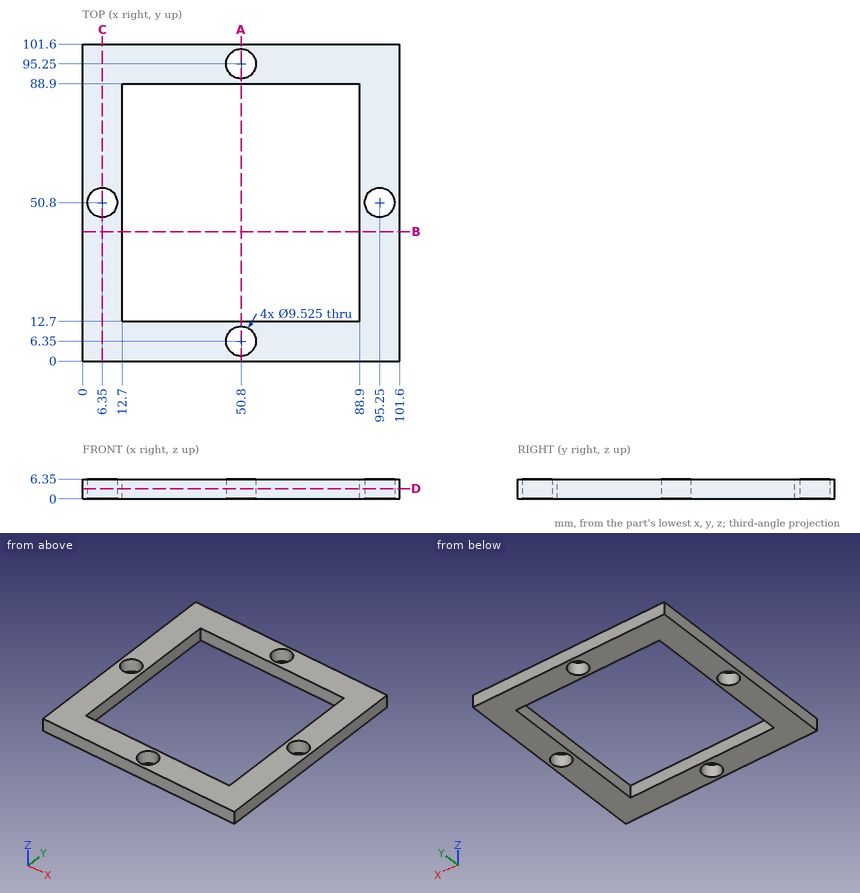
Could you check a few things on this drawing? It's one solid part, dimensions in mm from its lowest x, y, z. Coordinates: 2 decimals unless noted, no trailing zeros. Loops run counter-clockwise (first coordinate to the right, second up) from the corner with the lowest first, then second, coordinate; pieces in that order, holes last. Notation, with made-up numbers: (78.5, -7.5) - (124.5, -7.5) arc R22 cw to (124.5, 16.5) - close; hole circle Ø1 at (-20.5, 43.5). An arc over 180 degrees is marked (long way). Return JSON: item names as keys, results as strings. Group by question number.
Item 1: If we section it at A-A on x = 50.8: Write out the boundary of the cut face in (y, z), and give its area (3 significant figures).
Item 2: If we section it at C-C on x = 6.35: Write out the boundary of the cut face in (y, z), and give its area (3 significant figures).
Item 3: If we section it at B-B on y = 41.5: Write out the boundary of the cut face in (x, z), and give its area (3 significant figures).
Item 4: If we section it at D-D on z = 3.25: State how many separate pieces and enclosed holes the cut face has, and give its area (3 significant figures).
Item 5: Will this pin go through, and if not, where does the flat tip stop? P1, Ø5.5, axis at x = 50.8, y = 6.35, coming from the -Z side.
Item 6: I need wall thicknesses on line 1 (Y direction, x = 50.8, z = 4.5); line 2 (Y direction, x = 6.35, z = 2.25); line 3 (X direction, y = 44, z = 2.25). Which ranges of each line are inside material? Lowest first, please. Write a range as from..to.
Calculated:
{
 "1": {"outline": "(0, 0) - (1.59, 0) - (1.59, 6.35) - (0, 6.35) - close; (11.11, 0) - (12.7, 0) - (12.7, 6.35) - (11.11, 6.35) - close; (88.9, 0) - (90.49, 0) - (90.49, 6.35) - (88.9, 6.35) - close; (100.01, 0) - (101.6, 0) - (101.6, 6.35) - (100.01, 6.35) - close", "area": "40.3 mm^2"},
 "2": {"outline": "(0, 0) - (46.04, 0) - (46.04, 6.35) - (0, 6.35) - close; (55.56, 0) - (101.6, 0) - (101.6, 6.35) - (55.56, 6.35) - close", "area": "585 mm^2"},
 "3": {"outline": "(0, 0) - (12.7, 0) - (12.7, 6.35) - (0, 6.35) - close; (88.9, 0) - (101.6, 0) - (101.6, 6.35) - (88.9, 6.35) - close", "area": "161 mm^2"},
 "4": {"separate pieces": "1", "enclosed holes": "5", "area": "4,230 mm^2"},
 "5": {"P1": "passes through"},
 "6": {"line 1": "y = 0..1.59, 11.11..12.7, 88.9..90.49, 100.01..101.6", "line 2": "y = 0..46.04, 55.56..101.6", "line 3": "x = 0..12.7, 88.9..101.6"}
}
